Answer from the drawing. Dimensions are ordinates in mm from the lowest x, y and z of the part. Give positions to 0.01 mm unless a question says otherwise; leave off trailing zeros. Write each loop counter-clockwise with the first axis right and the second up, starting at its lowest first coordinate (ties: lowest second). Pieces come first, ordered by that corner, then holes. Notation, with made-up numbers: (33.5, 57.5) -> (61.5, 57.5) arc R11 ccw to (61.5, 73.5) -> close; hole circle Ø3 at (16, -17.75). An arc over 180 degrees is marked (long way). Write item = value, one per line.
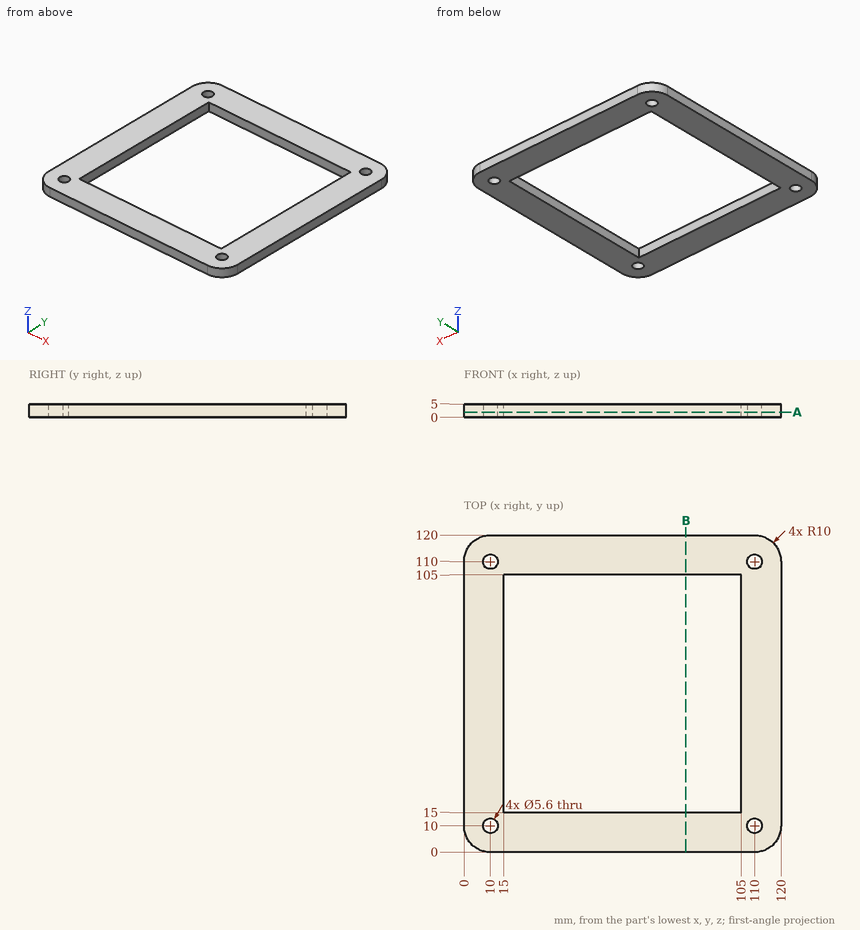
(1) Consider L1, parallel to Y at x = 110, z = 3.25; L2, parallel to Y at x = 39.5, z = 0.75. Determine where each line is inside the solid, lowest interval first.
Checks:
L1 = 0 to 7.2, 12.8 to 107.2, 112.8 to 120
L2 = 0 to 15, 105 to 120
(2) The part is cut by section A-A on z = 1.9. Determine the outline of the cut face in (x, y).
Checks:
outline = (0, 10) arc R10 ccw to (10, 0) -> (110, 0) arc R10 ccw to (120, 10) -> (120, 110) arc R10 ccw to (110, 120) -> (10, 120) arc R10 ccw to (0, 110) -> close; hole circle Ø5.6 at (10, 10); hole circle Ø5.6 at (10, 110); hole (15, 15) -> (105, 15) -> (105, 105) -> (15, 105) -> close; hole circle Ø5.6 at (110, 10); hole circle Ø5.6 at (110, 110)
(3) Given P1, Ø7.5, axis at x = 110, y = 10, coming from the -Z side, flat-ended and moving along its own axis, determine where the tip first touches the part or whether it passes through.
Checks:
P1 = 0
(4) The part is cut by section B-B on x = 84. Determine the outline of the cut face in (y, z).
Checks:
outline = (0, 0) -> (15, 0) -> (15, 5) -> (0, 5) -> close; (105, 0) -> (120, 0) -> (120, 5) -> (105, 5) -> close
